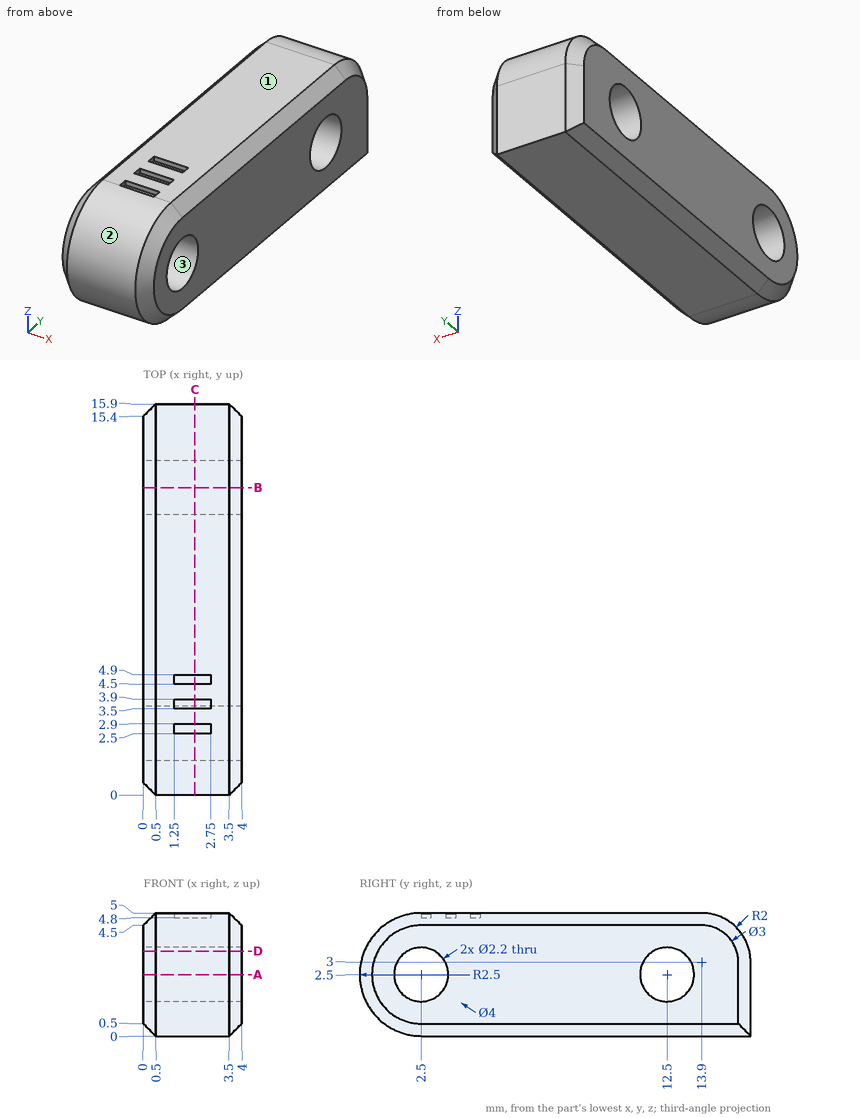
Part print with two shaded views. Sizes in mm from the minimum x, y, z corner. Round coordinates to 2 decimals unless told otherwise and drop trailing zeros. Write each loop counter-clockwise with the first axis right and the second up, starting at its lowest first coordinate (ties: lowest second). Pieces come first, ordered by that corner, then holes. Notation, with made-up numbers: M 45,67.25 L 80,67.25 A34 cw 80,105.25 Z; hole C -1.5,49.5 d11. An arc over 180 degrees is marked long. Put each result on its own line as item: value. Start each with the question number.
1) Pull direction Z, two halves, no side cores. Call the marked faces 1, 2 and 3: pulls with the +Z half, pulls with the -Z half, needs draft (parallel to the pull), parting line crosses it, or undercut.
2) Drill centre lines: probe 1 along Y at (x, z) = (0.9, 2.45); probe 2 along Z at (x, y) = (0.75, 2.5); probe 3 along Y at (x, z) = (2.4, 1.9). Where is each one in solid material? Low to high. Write a range as [from, to].
3) Saw through at C-C, the plane x = 2.1. Write the cut outline in (y, z), and give its area (3 significant figures).
4) Saw through at A-A, the plane z = 2.5. Write the cut outline in (x, y), and give its area (3 significant figures).
5) Saw through at D-D, the plane z = 3.45. Count the separate pieces of the cut face and the enclosed holes in it, and give its area (3 significant figures).
6) Saw through at B-B, the plane y = 12.5. Write the cut outline in (x, z).
Resolved:
1. face 1: pulls with the +Z half
1. face 2: parting line crosses it
1. face 3: undercut
2. probe 1: [0, 1.4], [3.6, 11.4], [13.6, 15.9]
2. probe 2: [0, 1.4], [3.6, 5]
2. probe 3: [0.07, 1.58], [3.42, 11.58], [13.42, 15.9]
3. outline: M 2.5,0 L 15.9,0 L 15.9,3 A2 ccw 13.9,5 L 4.9,5 L 4.9,4.8 L 4.5,4.8 L 4.5,5 L 3.9,5 L 3.9,4.8 L 3.5,4.8 L 3.5,5 L 2.9,5 L 2.9,4.8 L 2.5,4.8 L 2.5,5 A2.5 ccw Z; hole C 2.5,2.5 d2.2; hole C 12.5,2.5 d2.2
3. area: 68.1 mm²
4. outline: M 0,0.5 L 0.5,0 L 3.5,0 L 4,0.5 L 4,1.4 L 0,1.4 Z; M 0,3.6 L 4,3.6 L 4,11.4 L 0,11.4 Z; M 0,13.6 L 4,13.6 L 4,15.4 L 3.5,15.9 L 0.5,15.9 L 0,15.4 Z
4. area: 45.5 mm²
5. separate pieces: 3
5. enclosed holes: 0
5. area: 53.2 mm²
6. outline: M 0,0.5 L 0.5,0 L 3.5,0 L 4,0.5 L 4,1.4 L 0,1.4 Z; M 0,3.6 L 4,3.6 L 4,4.5 L 3.5,5 L 0.5,5 L 0,4.5 Z
